Design review of the part shown in the three views and the two pictorial views. Dimensions are in mm from the part's minimum x, y and z. A direction names the side the tool comes from. Round coordinates to 2 decimals unless told otherwise and drop trailing zeros. Loops run counter-clockwise (first coordinate to the right, second up) from the corner with the lowest first, then second, coordinate; pieces in that order, holes last. Notation, with made-up numbers: (15, 41) -> (70, 41) arc R26 cw to (70, 80) -> close; hole circle Ø10 at (65, -19.75). An arc over 180 degrees is marked (long way). Use a Markdown table: item, result. Add a question column.
1) Mouldability with a two-part tool opening along Z and no side actions: class the marked faces 1, 2 and 3 as released by +Z, released by -Z, zero draft, split by the parting line, or undercut.
2) For the marked faces 4, 5, 6 and 7, list the 3-axis set-ups (+Z, -Z, +X, -X, +Y, -Y) from which the entire face can be reached by the end or side of a thin tool; tool diameter is ignored.
3) Insertion check: pin 1 (3 mm diameter, centred on x = 11, z = 12.5, fed in from -Y); pin 2 (6.5 mm diameter, centred on x = 5, z = 8, fed in from +Y); pin 3 (9 mm diameter, centred on y = 42.5, z = 5.5, fed in from -X). Each pin has a flat end and moves straight along its axis. Give the tip position at first contact, or say it passes through.
4) Wall thickness on probe 1 along X at (y, z) = (29, 8) (3 decimals); probe 2 along Y at (x, z) = (17, 5); probe 3 along Z at (x, y) = (5, 20.5): over which ranges is each line inside the solid? List them lowest first.
5) Consider section B-B on z = 8. Give the boundary of the cut face in (x, y).
6) Consider section D-D on z = 4.5. Give the boundary of the cut face in (x, y).
7) Consider section A-A on y = 43. Give the boundary of the cut face in (x, z), plus the area to 3 significant figures.
8) Consider section C-C on x = 5. Give the boundary of the cut face in (y, z), plus the area to 3 significant figures.
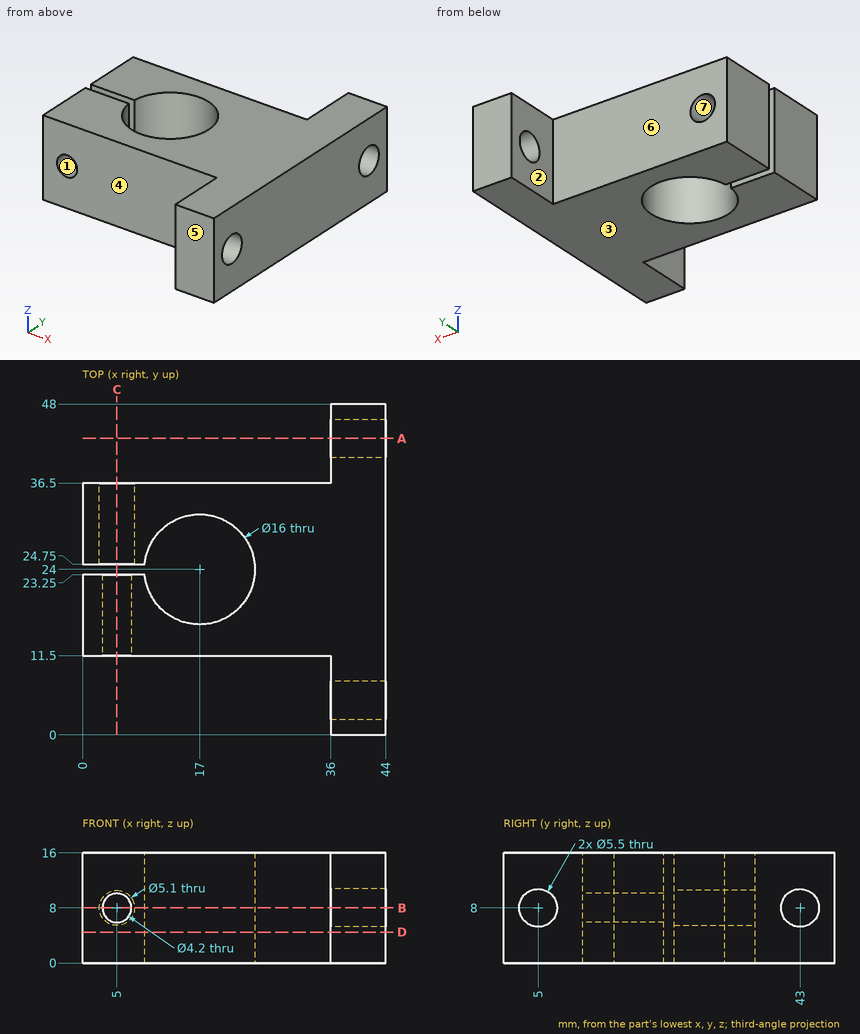
Result set:
| question | item | result |
|---|---|---|
| 1 | face 1 | undercut |
| 1 | face 2 | zero draft |
| 1 | face 3 | released by -Z |
| 2 | face 4 | +Z, -Z, -X, -Y |
| 2 | face 5 | +Z, -Z, +X, -X, -Y |
| 2 | face 6 | +Z, -Z, -X, +Y |
| 2 | face 7 | +Y |
| 3 | pin 1 | y = 11.5 |
| 3 | pin 2 | y = 36.5 |
| 3 | pin 3 | x = 36 |
| 4 | probe 1 | 0 to 2.45, 7.55 to 10.755, 23.245 to 44 |
| 4 | probe 2 | 11.5 to 16, 32 to 36.5 |
| 4 | probe 3 | 0 to 5.9, 10.1 to 16 |
| 5 | outline | (0, 11.5) -> (2.9, 11.5) -> (2.9, 23.25) -> (0, 23.25) -> close; (0, 24.75) -> (2.45, 24.75) -> (2.45, 36.5) -> (0, 36.5) -> close; (7.1, 11.5) -> (36, 11.5) -> (36, 7.75) -> (44, 7.75) -> (44, 40.25) -> (36, 40.25) -> (36, 36.5) -> (7.55, 36.5) -> (7.55, 24.75) -> (9.04, 24.75) arc R8 cw (long way) to (9.04, 23.25) -> (7.1, 23.25) -> close; (36, 0) -> (44, 0) -> (44, 2.25) -> (36, 2.25) -> close; (36, 45.75) -> (44, 45.75) -> (44, 48) -> (36, 48) -> close |
| 6 | outline | (0, 11.5) -> (36, 11.5) -> (36, 0) -> (44, 0) -> (44, 48) -> (36, 48) -> (36, 36.5) -> (0, 36.5) -> (0, 24.75) -> (9.04, 24.75) arc R8 cw (long way) to (9.04, 23.25) -> (0, 23.25) -> close |
| 7 | outline | (36, 0) -> (44, 0) -> (44, 5.25) -> (36, 5.25) -> close; (36, 10.75) -> (44, 10.75) -> (44, 16) -> (36, 16) -> close |
| 7 | area | 84.0 mm2 |
| 8 | outline | (11.5, 0) -> (23.25, 0) -> (23.25, 5.9) -> (11.5, 5.9) -> close; (11.5, 10.1) -> (23.25, 10.1) -> (23.25, 16) -> (11.5, 16) -> close; (24.75, 0) -> (36.5, 0) -> (36.5, 5.45) -> (24.75, 5.45) -> close; (24.75, 10.55) -> (36.5, 10.55) -> (36.5, 16) -> (24.75, 16) -> close |
| 8 | area | 267 mm2 |
